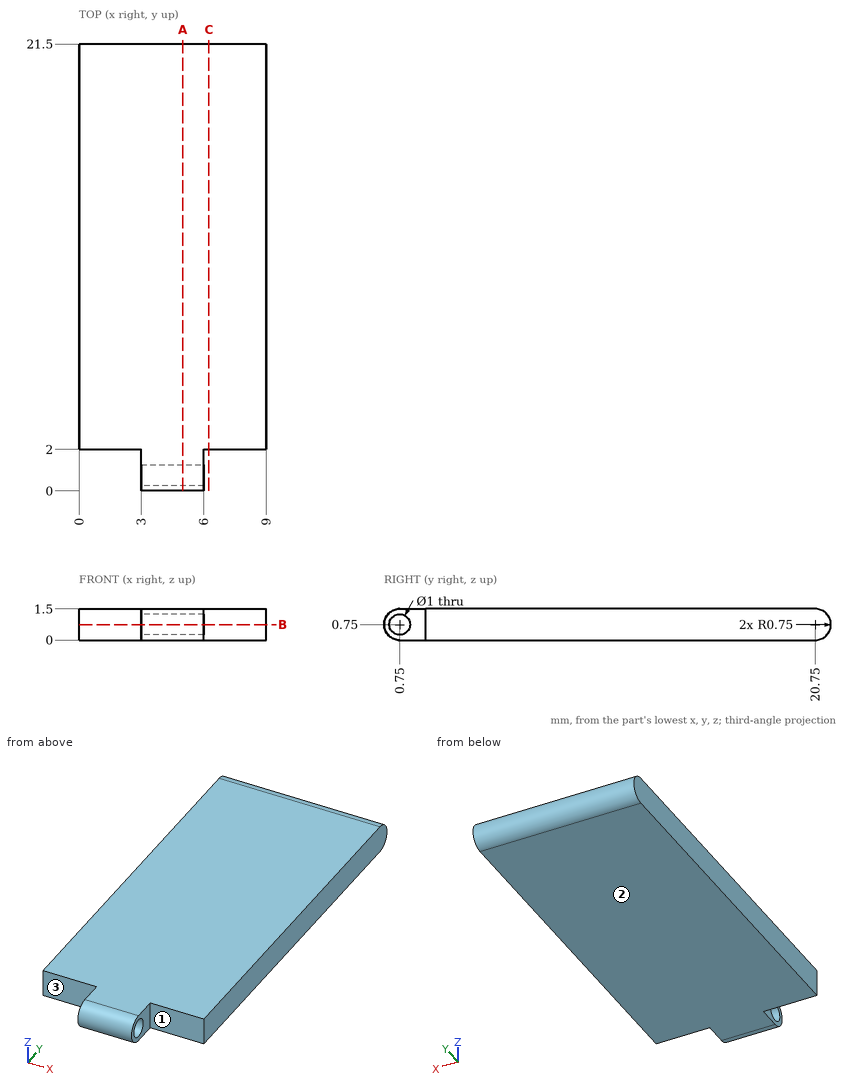
Source: three-view drawing plus pictorial views. Frame: mm from the lowest corner of the part. A direction names the side the tool comes from. Give positions to 0.01 mm unless a question says otherwise; leave off trailing zeros. Order: outer loops, then holes, each group sorted by start corner. A loop starts at its lowest first (then second) coordinate and runs counter-clockwise, first axis right, second up.
1. Section B-B on z = 0.75. Return the cut outline in (x, y).
Derived:
outline: (0, 2) - (3, 2) - (3, 1.25) - (6, 1.25) - (6, 2) - (9, 2) - (9, 21.5) - (0, 21.5) - close; (3, 0) - (6, 0) - (6, 0.25) - (3, 0.25) - close
2. Pin query (flat end, axial travel): pin 1 (0.8 mm diameter, centred on x = 1, z = 1, fed in from -Y). Return the tip coordinate at first contact, or that it passes through.
Derived:
pin 1: stops at y = 2
3. Reachability of the marked faces 1, 2 and 3 from +Z, -Z, +X, -X, +Y, -Y: full face, straight path, thin tool, end or side. Return the list, or none.
Derived:
face 1: +Z, -Z, +X, -Y
face 2: -Z, +X, -X, +Y, -Y
face 3: +Z, -Z, -X, -Y
4. Section C-C on x = 6.25. Return the cut outline in (y, z).
Derived:
outline: (2, 0) - (20.75, 0) arc R0.75 ccw to (20.75, 1.5) - (2, 1.5) - close
5. Section A-A on x = 5. Return the cut outline in (y, z), and give its area (3 significant figures).
Derived:
outline: (0.75, 0) - (20.75, 0) arc R0.75 ccw to (20.75, 1.5) - (0.75, 1.5) arc R0.75 ccw to start; hole circle Ø1 at (0.75, 0.75)
area: 31.0 mm2
6. Material intervals for L1, parallel to Y at x = 4.55, z = 0.75; L2, parallel to Z at x = 4.35, y = 0.75; L3, parallel to Y at x = 1, z = 0.8, sorted ascending.
Derived:
L1: y = 0 to 0.25, 1.25 to 21.5
L2: z = 0 to 0.25, 1.25 to 1.5
L3: y = 2 to 21.5
